Check sheet for the modelled part. Datum: model origin and axes. Units: mm. Give positions to 0.01 mm unless a question says otherwise; leave off trailing zeros. Order: outer loops, then holes, each group sorted by start corner. A loop starts at its lowest first (then second) coordinate and runs counter-clockwise, first axis right, second up.
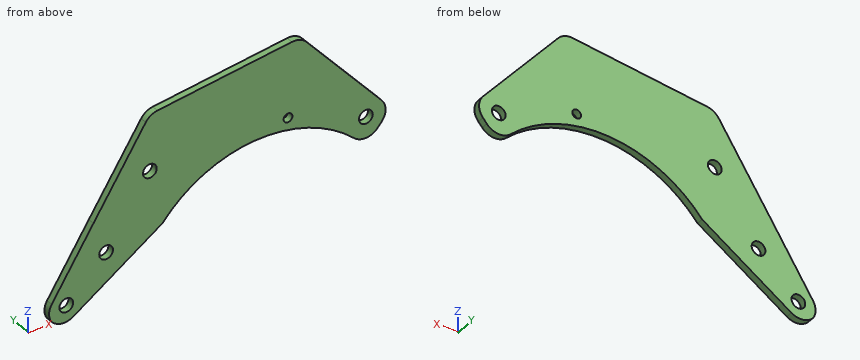
from build123d import *

# Parameters (mm, degrees)
SKETCH1_R           = 3.175
SKETCH1_R_2         = 2.032
BOSS_EXTRUDE1_DEPTH = 3.175
FILLET1_R           = 7.62


with BuildPart() as part:
    # Sketch1 → Boss-Extrude1 (new body)
    # profile 1 of 2: a face of its own
    with BuildSketch(Plane(origin=(0, 0, 0), x_dir=(1, 0, 0), z_dir=(0, 1, 0))):
        with BuildLine():
            Line((105.591118199, -28.343622072), (94.077776645, -14.794770967))
            ThreePointArc((94.077776645, -14.794770967), (47.065246085, -36.873172811), (0.097776645, -14.699073687))
            Line((0.097776645, -14.699073687), (-31.782789553, -26.688950722))
            Line((-31.782789553, -26.688950722), (-5.708312831, -67.169135043))
            Line((-5.708312831, -67.169135043), (63.939848964, -76.376354726))
            Line((63.939848964, -76.376354726), (105.591118199, -28.343622072))
        make_face()
        with Locations(Location((-5.708312831, -41.020609427, 0), (0, 0, 270))):
            Circle(SKETCH1_R, mode=Mode.SUBTRACT)
        with Locations(Location((58.097885383, -41.467741904, 0), (0, 0, 270))):
            Circle(SKETCH1_R_2, mode=Mode.SUBTRACT)
        with Locations(Location((94.077776645, -28.343622072, 0), (0, 0, 270))):
            Circle(SKETCH1_R, mode=Mode.SUBTRACT)
    # profile 2 of 2: a face of its own
    with BuildSketch(Plane(origin=(0, 0, 0), x_dir=(1, 0, 0), z_dir=(0, 1, 0))):
        Polygon((-31.782789553, -26.688950722), (0.097776645, -14.699073687), (-47.44057022, 17.052204331), (-53.745234427, 7.612794876), align=None)
        with Locations(Location((-25.919844617, -11.116586696, 0), (0, 0, 270))):
            Circle(SKETCH1_R, mode=Mode.SUBTRACT)
        with Locations(Location((-44.331222359, 6.381446612, 0), (0, 0, 270))):
            Circle(SKETCH1_R, mode=Mode.SUBTRACT)
    extrude(amount=BOSS_EXTRUDE1_DEPTH)

    # Fillet1
    # the kernel refuses this fillet: 7.62 mm, written as the material it takes off along each edge
    with BuildSketch(Plane(origin=(94.077776645, -21.209715088, 14.794770967), x_dir=(0.6475445193715758, 0, 0.7620276211738226), z_dir=(0, 1, 0))) as fillet1_piece_1:
        with BuildLine():
            CenterArc((8.483886035, -7.62), FILLET1_R, 90, 92.490451597)
            ThreePointArc((0.871083301, -7.951111055), (0.566092443, -3.961253046), (0, 0))
            Line((0, 0), (8.483886035, 0))
        make_face()
    extrude(amount=45.594430177, mode=Mode.SUBTRACT)
    with BuildSketch(Plane(origin=(105.591118199, -16.352843569, 28.343622072), x_dir=(-0.6551362182138352, 0, 0.755510777940642), z_dir=(0, 1, 0))) as fillet1_piece_2:
        with BuildLine():
            CenterArc((FILLET1_R * 0.858416985261, -FILLET1_R), FILLET1_R, 90, 81.28670352)
            Line((-FILLET1_R * 0.130041772231, -FILLET1_R * 0.848509786661), (0, 0))
            Line((0, 0), (FILLET1_R * 0.858416985261, 0))
        make_face()
    extrude(amount=35.880687138, mode=Mode.SUBTRACT)
    with BuildSketch(Plane(origin=(63.939848964, -10.25750483, 76.376354726), x_dir=(0.6551362182138344, 0, -0.7555107779406426), z_dir=(0, 1, 0))) as fillet1_piece_3:
        with BuildLine():
            CenterArc((FILLET1_R * 0.538451697109, FILLET1_R), FILLET1_R, 213.399362726, 56.600637274)
            Line((-FILLET1_R * 0.296402288845, FILLET1_R * 0.449528545576), (0, 0))
            Line((0, 0), (FILLET1_R * 0.538451697109, 0))
        make_face()
    extrude(amount=23.69000966, mode=Mode.SUBTRACT)
    with BuildSketch(Plane(origin=(-5.708312831, -8.81900629, 67.169135043), x_dir=(0.9913749712814725, 0, 0.13105596635277514), z_dir=(0, 1, 0))) as fillet1_piece_4:
        with BuildLine():
            CenterArc((FILLET1_R * 0.462939962752, FILLET1_R), FILLET1_R, 220.317392239, 49.682607761)
            Line((-FILLET1_R * 0.29953199758, FILLET1_R * 0.352978740916), (0, 0))
            Line((0, 0), (FILLET1_R * 0.462939962752, 0))
        make_face()
    extrude(amount=20.813012581, mode=Mode.SUBTRACT)
    with BuildSketch(Plane(origin=(-47.44057022, -19.05, -17.052204331), x_dir=(0.8315732701891384, 0, 0.5554150666906167), z_dir=(0, 1, 0))) as fillet1_piece_5:
        with BuildLine():
            CenterArc((FILLET1_R, -FILLET1_R), FILLET1_R, 90, 90)
            Line((0, -FILLET1_R), (0, 0))
            Line((0, 0), (FILLET1_R, 0))
        make_face()
    extrude(amount=41.275, mode=Mode.SUBTRACT)
    with BuildSketch(Plane(origin=(-53.745234427, -12.458754806, -7.612794876), x_dir=(0.5392161516528728, 0, 0.8421674072277234), z_dir=(0, 1, 0))) as fillet1_piece_6:
        with BuildLine():
            CenterArc((FILLET1_R * 0.654002876977, FILLET1_R), FILLET1_R, 203.630396876, 66.369603124)
            Line((-FILLET1_R * 0.262147328242, FILLET1_R * 0.599164869956), (0, 0))
            Line((0, 0), (FILLET1_R * 0.654002876977, 0))
        make_face()
    extrude(amount=28.092509613, mode=Mode.SUBTRACT)


solid = part.part
1) Section check B-B, the plane y = 2.3. State how many separate pieces and enclosed holes the cut face has, then the cut area to 3 significant figures.
Recorded:
separate pieces: 1
enclosed holes: 5
area: 5,480 mm2
2) Depth check by flat-ended pin: pin 1 Ø1.5 at (y, z) = (0.5, -4) entering from +X; pin 2 Ø7.5 at (x, z) = (-25.92, 11.12) entering from +Y (3 decimals); pin 3 Ø1 at (x, y) = (47.5, 2.5) entering from +Z; pin 4 Ø4 at (x, z) = (-5.71, 41.02) entering from -Y. Enter the tip coordinate at first touch or a pass-through.
Recorded:
pin 1: stops at x = -26.78
pin 2: stops at y = 3.175
pin 3: stops at z = 74.27
pin 4: passes through
3) Material ranges on L1, parallel to X at y = 2.2, z = 41; L2, parallel to X at y = 2.55, z = 8.5; L3, parallel to Z at x = -4, y = 1.25, recorded low to high.
Recorded:
L1: x = -22.56 to -8.88, -2.53 to 56.12, 60.08 to 94.62
L2: x = -43.43 to -27.72, -24.12 to -9.18
L3: z = 11.96 to 38.34, 43.7 to 67.17
4) Section check C-C, the plane x = -19.5. Record the cut outline in (y, z) (3 decimals), then the cut area to 3 significant figures.
Recorded:
outline: (0, 1.61) - (3.175, 1.61) - (3.175, 45.758) - (0, 45.758) - close
area: 140 mm2
5) Section check A-A, the plane z = -7. Record the cut outline in (x, y) (3 decimals), then the cut area to 3 significant figures.
Recorded:
outline: (-52.243, 0) - (-47.445, 0) - (-47.445, 3.175) - (-52.243, 3.175) - close; (-41.217, 0) - (-32.39, 0) - (-32.39, 3.175) - (-41.217, 3.175) - close
area: 43.3 mm2
6) Section check D-D, the plane z = 52.5. Record the cut outline in (x, y) (3 decimals), then the cut area to 3 significant figures.
Recorded:
outline: (-15.157, 0) - (84.644, 0) - (84.644, 3.175) - (-15.157, 3.175) - close
area: 317 mm2
